Here's how the part is built. I have some questions about the finished solid (model axes, mm). Face numbers are marked on the shaded views. A direction names the side the tool comes from. Coordinates: 2 decimals unless noted, no trailing zeros. Write each loop counter-clockwise with the first axis right and the second up, starting at its lowest first coordinate (ties: lowest second). Pieces come first, ordered by that corner, then holes.
Item 1: If I drill on line 1 (X direction, y = 5, z = 97); line 2 (Z direction, x = 10, y = -10.5); line 3 (Y direction, x = -66.5, z = -26), over which ranges is the centre line in solid material (lowest first)?
Item 2: If we section it at D-D (x = 12): Please give me the cut outline in (y, z), then the cut area to 3 significant figures.
Item 3: If we section it at B-B (z = 112): Please give me the cut outline in (x, y), then the cut area to 3 significant figures.
Item 4: If we section it at C-C (y = 12.5): Please give me the cut outline in (x, z), then the cut area to 3 significant figures.
Item 5: I'm going to push flat-ended pins straight in: pin 1 Ø8 at (y, z) = (3, 78.5) entering from +X; pin 2 Ø9 at (x, z) = (-54, -30) entering from -Y; pin 3 Ø12 at (y, z) = (8, 75.5) entering from -X; pin 4 Ø7.5 at (x, z) = (-63.5, 38) entering from +Y. Where does each tip first touch, or does it pass through?
Item 6: If we section it at A-A (x = -44.5): Please give me the cut outline in (y, z), then the cut area to 3 significant figures.
Item 7: For the marked faces 1, 2 and 3, which set-ups out of +Z, -Z, +X, -X, +Y, -Y let a thin tool reach every point of the face, with its end or its side?
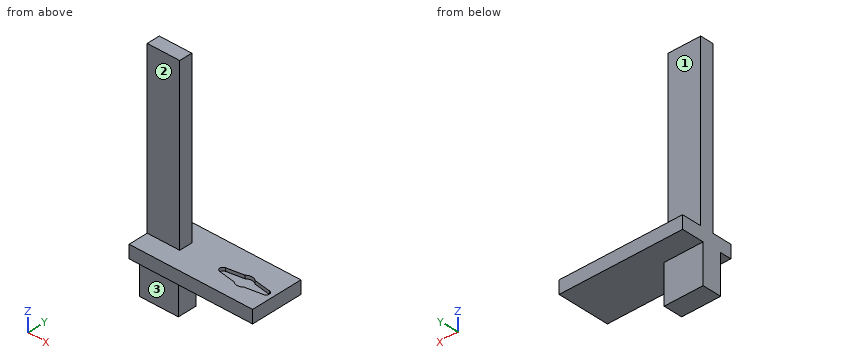
from build123d import *

# Parameters (mm, degrees)
SKETCH3_W            = 45
SKETCH3_H            = 15
BOSS_EXTRUDE1_DEPTH  = 10
CUT_EXTRUDE1_DEPTH   = 2.5
SKETCH11_W           = 45
SKETCH11_H           = 10
BOSS_EXTRUDE5_DEPTH  = 10
SKETCH14_W           = 45
SKETCH14_H           = 10
BOSS_EXTRUDE7_DEPTH  = 15
SKETCH20_W           = 10
SKETCH20_H           = 40
BOSS_EXTRUDE10_DEPTH = 50
SKETCH21_W           = 25
SKETCH21_H           = 10
BOSS_EXTRUDE11_DEPTH = 130
SKETCH22_W           = 30
SKETCH22_H           = 6
BOSS_EXTRUDE12_DEPTH = 30
SKETCH23_W           = 30
SKETCH23_H           = 30
BOSS_EXTRUDE13_DEPTH = 8.5


with BuildPart() as part:
    # Sketch3 → Boss-Extrude1 (new body)
    with BuildSketch(Plane.XY):
        with Locations((-0.138845539, 0.05888455)):
            Rectangle(SKETCH3_W, SKETCH3_H)
    extrude(amount=-BOSS_EXTRUDE1_DEPTH)

    # Sketch2 → Cut-Extrude1 (cut)
    with BuildSketch(Plane.XY):
        with BuildLine():
            Line((-16.888114198, 2.469689731), (-3.968626967, 4.5))
            ThreePointArc((-3.968626967, 4.5), (0, 6), (3.968626967, 4.5))
            Line((3.968626967, 4.5), (16.888114198, 2.469689731))
            ThreePointArc((16.888114198, 2.469689731), (19, 0), (16.888114198, -2.469689731))
            Line((16.888114198, -2.469689731), (3.968626967, -4.5))
            ThreePointArc((3.968626967, -4.5), (0, -6), (-3.968626967, -4.5))
            Line((-3.968626967, -4.5), (-16.888114198, -2.469689731))
            ThreePointArc((-16.888114198, -2.469689731), (-19, 0), (-16.888114198, 2.469689731))
        make_face()
    extrude(amount=-CUT_EXTRUDE1_DEPTH, mode=Mode.SUBTRACT)

    # Sketch11 → Boss-Extrude5 (add)
    with BuildSketch(Plane.XZ.offset(7.44111545)):
        with Locations((-0.138845539, -5)):
            Rectangle(SKETCH11_W, SKETCH11_H)
    extrude(amount=BOSS_EXTRUDE5_DEPTH)

    # Sketch14 → Boss-Extrude7 (add)
    with BuildSketch(Plane(origin=(0, 7.55888455, 0), x_dir=(1, 0, 0), z_dir=(0, 1, 0))):
        with Locations((-0.138845539, 5)):
            Rectangle(SKETCH14_W, SKETCH14_H)
    extrude(amount=BOSS_EXTRUDE7_DEPTH)

    # Sketch20 → Boss-Extrude10 (add)
    with BuildSketch(Plane.ZY.offset(22.638845539)):
        with Locations((-5, 2.55888455)):
            Rectangle(SKETCH20_W, SKETCH20_H)
    extrude(amount=BOSS_EXTRUDE10_DEPTH)

    # Sketch21 → Boss-Extrude11 (add)
    with BuildSketch(Plane.XY):
        with Locations((-60.138845539, 2.55888455)):
            Rectangle(SKETCH21_W, SKETCH21_H)
    extrude(amount=BOSS_EXTRUDE11_DEPTH)

    # Sketch22 → Boss-Extrude12 (add)
    with BuildSketch(Plane(origin=(0, 0, -10), x_dir=(-1, 0, 0), z_dir=(0, 0, -1))):
        with Locations((57.638845539, 2.55888455)):
            Rectangle(SKETCH22_W, SKETCH22_H)
    extrude(amount=BOSS_EXTRUDE12_DEPTH)

    # Sketch23 → Boss-Extrude13 (add)
    with BuildSketch(Plane.XZ.offset(0.44111545)):
        with Locations((-57.638845539, -25)):
            Rectangle(SKETCH23_W, SKETCH23_H)
    extrude(amount=BOSS_EXTRUDE13_DEPTH)


solid = part.part
Answer list:
1. line 1: x = -72.64 to -47.64
1. line 2: z = -10 to 0
1. line 3: y = -8.94 to 5.56
2. outline: (-17.44, -10) - (22.56, -10) - (22.56, 0) - (3.24, 0) - (3.24, -2.5) - (-3.24, -2.5) - (-3.24, 0) - (-17.44, 0) - close
2. area: 384 mm2
3. outline: (-72.64, -2.44) - (-47.64, -2.44) - (-47.64, 7.56) - (-72.64, 7.56) - close
3. area: 250 mm2
4. outline: (-72.64, -10) - (22.36, -10) - (22.36, 0) - (-72.64, 0) - close
4. area: 950 mm2
5. pin 1: stops at x = -47.64
5. pin 2: stops at y = -8.94
5. pin 3: stops at x = -72.64
5. pin 4: stops at y = 7.56
6. outline: (-17.44, -10) - (-8.94, -10) - (-8.94, -40) - (5.56, -40) - (5.56, -10) - (22.56, -10) - (22.56, 0) - (-17.44, 0) - close
6. area: 835 mm2
7. face 1: +Z, +X, -X, +Y
7. face 2: +Z, +X, -X, -Y
7. face 3: -Z, +X, -X, -Y
